The model under review builds one solid part; all positions refer to its coordinate system, in mm. Face numbers are marked on the shaded views. Coordinates: 2 decimals unless noted, no trailing zeros. Order: outer loops, then holes, each group sorted by start corner. A loop starts at its lowest first (then second) coordinate and runs counter-clockwise, first axis right, second up.
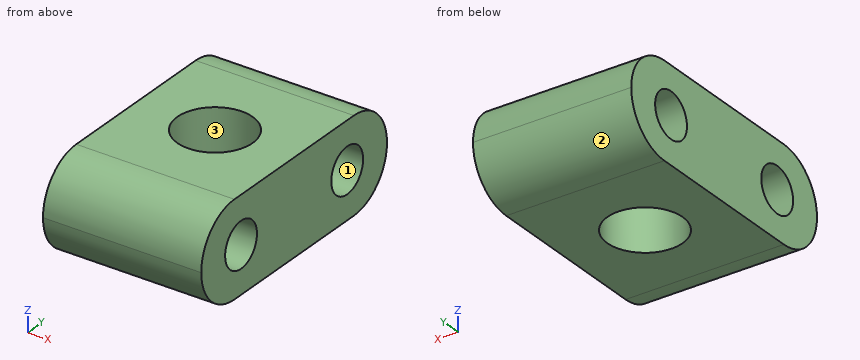
Autodesk Inventor part; units mm, degrees
ref_plane "YZ Plane" through (0, 0, 0) normal (1, 0, 0) x (0, 1, 0)
ref_plane "XZ Plane" through (0, 0, 0) normal (0, 1, 0) x (-1, 0, 0)
ref_plane "XY Plane" through (0, 0, 0) normal (0, 0, 1) x (1, 0, 0)
sketch "Sketch2" plane through (0, 0, 0) normal (1, 0, 0) x (0, 1, 0)
  line L0 (35, 12.5) -> (35, -12.5)
  line L1 (35, -12.5) -> (-35, -12.5)
  line L2 (-35, -12.5) -> (-35, 12.5)
  line L3 (-35, 12.5) -> (35, 12.5)
  point P0 (0, 0)
  dimension "d11" = 25
  dimension "d12" = 70
  dimension "d13" = 35
  dimension "d14" = 12.5
extrude "Extrusion2" add sketch "Sketch2" along normal blind 42
full round fillet "Full Round Fillet1" first side at (14, 11.6667, 12.5) centre faces at (14, 35, -4.1667) second side at (14, -11.6667, -12.5)
full round fillet "Full Round Fillet2" first side at (28, 3.3334, 12.5) centre faces at (14, -35, 4.1667) second side at (14, -15.8333, -12.5)
sketch "Sketch3" plane through (42, 22.5, -12.5) normal (0, 0, -1) x (-1, 0, 0)
  circle A0 centre (21, -22.5) radius 10
  line L0 (42, -45) -> (42, 0)
  point P0 (42, -22.5)
  point P1 (42, -22.5)
  dimension "d15" = 20
  dimension "d16" = 21
sketch "Sketch4" plane through (42, 0, 0) normal (1, 0, 0) x (0, 0, -1)
  circle A0 centre (0, -20) radius 6
  circle A1 centre (0, 20) radius 6
  point P0 (0, 0)
  dimension "d17" = 12
  dimension "d18" = 12
  dimension "d31" = 40
  dimension "d32" = 20
extrude "Extrusion3" cut sketch "Sketch3" against normal blind 42
extrude "Extrusion4" cut sketch "Sketch4" against normal blind 42
thread "Thread1"
thread "Thread2"
thread "Thread4"
properties part number "Junção Fuso" material "Steel AISI 1050"
(1) We need section A-A, the plane x = 21. Count the separate pieces of the cut face and the enclosed holes in it, and give its area (3 significant figures).
A:
separate pieces: 2
enclosed holes: 2
area: 890 mm2
(2) We need section B-B, the plane y = 0. Write out the cut boundary in (x, z).
A:
outline: (0, -12.5) - (11, -12.5) - (11, 12.5) - (0, 12.5) - close; (31, -12.5) - (42, -12.5) - (42, 12.5) - (31, 12.5) - close
(3) Wall thickness on probe 1 along Y at (x, z) = (33, -3); probe 2 along Y at (x, z) = (21, 5); probe 3 along Y at (x, z) = (24, 0): over which ranges is each line inside the solid? List them lowest first.
A:
probe 1: y = -34.63 to -25.2, -14.8 to 14.8, 25.2 to 34.63
probe 2: y = -33.96 to -23.32, -16.68 to -10, 10 to 16.68, 23.32 to 33.96
probe 3: y = -35 to -26, -14 to -9.54, 9.54 to 14, 26 to 35
(4) We need section C-C, the plane z = -3.25. Write out the cut boundary in (x, y), and give its area (3 significant figures).
A:
outline: (0, -34.57) - (42, -34.57) - (42, -25.04) - (0, -25.04) - close; (0, -14.96) - (42, -14.96) - (42, 14.96) - (0, 14.96) - close; (0, 25.04) - (42, 25.04) - (42, 34.57) - (0, 34.57) - close; hole circle Ø20 at (21, 0)
area: 1,740 mm2
(5) Draft analysis for pull direction Z (two halves, no side actions). For the marked faces 1, 2 and 3, state which applies: released by +Z, released by -Z, zero draft, split by the parting line, or undercut.
A:
face 1: undercut
face 2: released by -Z
face 3: zero draft
